from build123d import *

# Parameters (mm, degrees)
F0_W     = 45
F0_H     = 35
F1_DEPTH = 35
F2_W     = 40
F2_H     = 30
F3_DEPTH = 30
F4_W     = 45
F4_H     = 35
F4_W_2   = 42
F4_H_2   = 32
F5_DEPTH = 10
F6_R     = 0.3


with BuildPart() as f1:
    # F0 (on Top) → F1 (new body)
    with BuildSketch(Plane.XY):
        Rectangle(F0_W, F0_H)
    extrude(amount=F1_DEPTH)

    # F2 (on face) → F3 (cut)
    with BuildSketch(Plane.XY.offset(35)):
        Rectangle(F2_W, F2_H)
    extrude(amount=-F3_DEPTH, mode=Mode.SUBTRACT)

    # F4 (on face) → F5 (cut)
    with BuildSketch(Plane.XY.offset(35)):
        Rectangle(F4_W, F4_H)
        Rectangle(F4_W_2, F4_H_2, mode=Mode.SUBTRACT)
    extrude(amount=-F5_DEPTH, mode=Mode.SUBTRACT)

    # F6
    f6_edges = [f1.edges().sort_by_distance(p)[0] for p in [
        (-22.5, 17.5, 12.5),
        (22.5, 17.5, 12.5),
        (22.5, -17.5, 12.5),
        (-22.5, -17.5, 12.5),
        (-21, -16, 30),
        (21, -16, 30),
        (21, 16, 30),
        (-21, 16, 30),
        (-20, 15, 20),
        (20, 15, 20),
        (20, -15, 20),
        (-20, -15, 20),
    ]]
    fillet(f6_edges, radius=F6_R)


solid = f1.part
Could you check a few things on this model? Use its own coordinates, in mm. A direction names the side the tool comes from. Give positions to 0.01 mm unless a question says otherwise; leave off trailing zeros. Order: outer loops, then holes, each group sorted by start corner. A loop starts at its lowest first (then second) coordinate and runs counter-clockwise, first axis right, second up. Notation, with made-up numbers: (24.5, -38.5) - (80.5, -38.5) arc R23 ccw to (80.5, -23.5) - close; hole circle Ø5 at (37.5, 84). An arc over 180 degrees is marked (long way). One line per question, with ' | ' between items. Start each with the question number.
Item 1: I need wall thicknesses on probe 1 along Y at (x, z) = (9, 16); probe 2 along X at (y, z) = (8, 19.5); probe 3 along Y at (x, z) = (14, 25.5). Which ranges of each line are inside material? Lowest first, please. Write a range as [from, to].
Item 2: Thinking about a two-plate mould opening in Y: for faces 4 (the flat face through (-21, 0, 30)), 5 (the flat face through (-20, 0, 20)), 6 (the flat face through (0, 17.5, 12)), which applies, pulls with the +Y half, pulls with the -Y half, needs draft (parallel to the pull), parting line crosses it, or undercut?
Item 3: I want a section at C-C on x = 0.5. Write out the boundary of the cut face in (y, z), then the cut area to 3 significant figures.
Item 4: I want a section at A-A on z = 18. Write out the boundary of the cut face in (x, y), then the cut area to 3 significant figures.
Item 5: For faces 1 (the flat face through (-2, -17, 25)), 2 (the flat face through (0, 16, 30)), 3 (the flat face through (21, 0, 30)), which set-ups out of +Z, -Z, +X, -X, +Y, -Y let a thin tool reach every point of the face, with its end or its side?
Item 6: I want a section at D-D on z = 30. Write out the boundary of the cut face in (x, y).
Item 7: I'm going to push flat-ended pins straight in: pin 1 Ø1.5 at (x, y) = (8.5, -11.5) entering from +Z; pin 2 Ø11 at (y, z) = (-5, 32) entering from +X; pin 3 Ø8 at (y, z) = (0.5, 32.5) entering from -X. Where does each tip first touch, or does it pass through?
Item 8: I want a section at B-B on y = -13. Write out the boundary of the cut face in (x, z).
Verdict:
1) probe 1: [-17.5, -15], [15, 17.5] | probe 2: [-22.5, -20], [20, 22.5] | probe 3: [-16, -15], [15, 16]
2) face 4: needs draft | face 5: undercut | face 6: pulls with the +Y half
3) outline: (-17.5, 0) - (17.5, 0) - (17.5, 25) - (16, 25) - (16, 35) - (15, 35) - (15, 5) - (-15, 5) - (-15, 35) - (-16, 35) - (-16, 25) - (-17.5, 25) - close | area: 295 mm^2
4) outline: (-22.5, -17.2) arc R0.3 ccw to (-22.2, -17.5) - (22.2, -17.5) arc R0.3 ccw to (22.5, -17.2) - (22.5, 17.2) arc R0.3 ccw to (22.2, 17.5) - (-22.2, 17.5) arc R0.3 ccw to (-22.5, 17.2) - close; hole (-20, -14.7) arc R0.3 ccw to (-19.7, -15) - (19.7, -15) arc R0.3 ccw to (20, -14.7) - (20, 14.7) arc R0.3 ccw to (19.7, 15) - (-19.7, 15) arc R0.3 ccw to (-20, 14.7) - close | area: 375 mm^2
5) face 1: +Z | face 2: +Z, +X, -X, +Y | face 3: +Z, +X, +Y, -Y
6) outline: (-21, -15.7) arc R0.3 ccw to (-20.7, -16) - (20.7, -16) arc R0.3 ccw to (21, -15.7) - (21, 15.7) arc R0.3 ccw to (20.7, 16) - (-20.7, 16) arc R0.3 ccw to (-21, 15.7) - close; hole (-20, -14.7) arc R0.3 ccw to (-19.7, -15) - (19.7, -15) arc R0.3 ccw to (20, -14.7) - (20, 14.7) arc R0.3 ccw to (19.7, 15) - (-19.7, 15) arc R0.3 ccw to (-20, 14.7) - close
7) pin 1: z = 5 | pin 2: x = 21 | pin 3: x = -21
8) outline: (-22.5, 0) - (22.5, 0) - (22.5, 25) - (21, 25) - (21, 35) - (20, 35) - (20, 5) - (-20, 5) - (-20, 35) - (-21, 35) - (-21, 25) - (-22.5, 25) - close
